Print and shaded views of the part. All mm, measured from the part's lowest x, y and z. Round coordinates to 2 decimals unless told otherwise and drop trailing zeros. Loops run counter-clockwise (first coordinate to the right, second up) from the corner with the lowest first, then second, coordinate; pieces in that order, holes last. Notation, with made-up numbers: (8, -13.75) -> (64, -13.75) arc R25 cw to (64, 6.25) -> close; hole circle Ø2 at (-33, 22). An arc over 180 degrees is marked (long way). Answer as CSV lines item,"result".
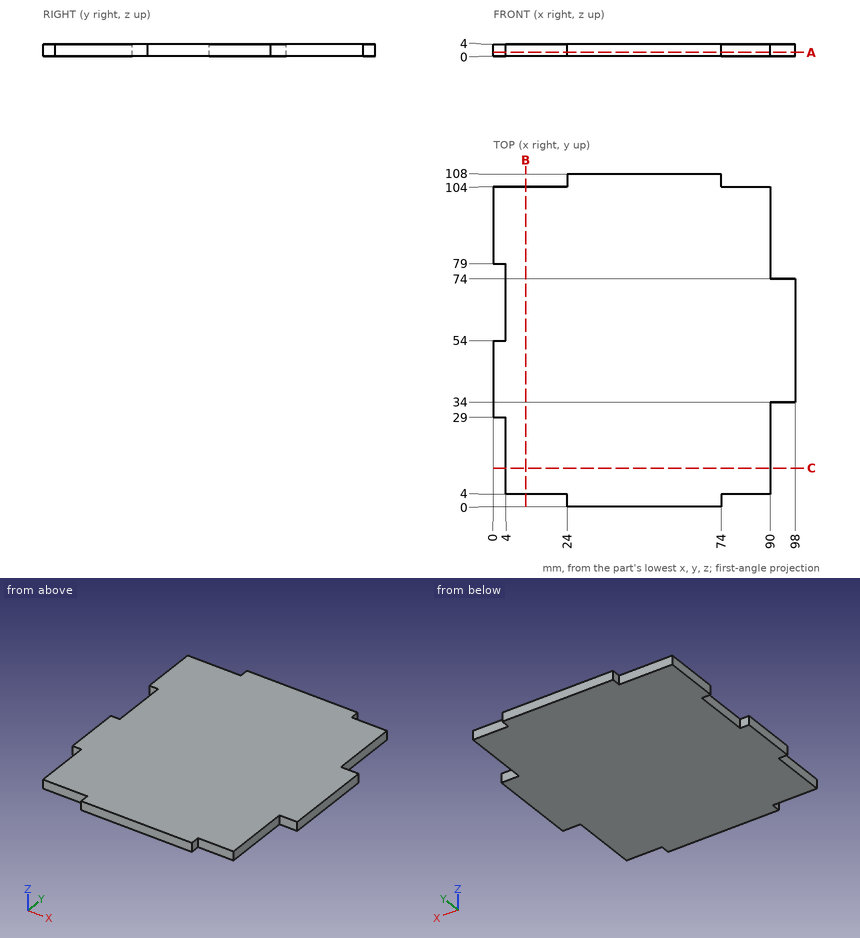
Q1. Slice it at C-C, the plane y = 12.5. Give the cut face in (x, z), and give its area (3 significant figures).
Results:
outline,"(4, 0) -> (90, 0) -> (90, 4) -> (4, 4) -> close"
area,"344 mm2"
Q2. Drop flat-ended pins along their axis: pin 1 Ø10 at (x, y) = (62, 78.5) entering from -Z; pin 2 Ø1.2 at (x, z) = (1, 1.5) entering from -Y; pin 3 Ø1.2 at (y, z) = (2.5, 1.5) entering from -X; pin 4 Ø2 at (x, z) = (78.5, 2) entering from -Y. Give the stop position or say it passes through.
Results:
pin 1,"z = 0"
pin 2,"y = 29"
pin 3,"x = 24"
pin 4,"y = 4"
Q3. Slice it at B-B, the plane x = 10.5. Give the cut face in (y, z), and give its area (3 significant figures).
Results:
outline,"(4, 0) -> (104, 0) -> (104, 4) -> (4, 4) -> close"
area,"400 mm2"
Q4. Slice it at A-A, the plane z = 1.25. Give the cut face in (x, y), and give its area (3 significant figures).
Results:
outline,"(0, 29) -> (4, 29) -> (4, 4) -> (24, 4) -> (24, 0) -> (74, 0) -> (74, 4) -> (90, 4) -> (90, 34) -> (98, 34) -> (98, 74) -> (90, 74) -> (90, 104) -> (74, 104) -> (74, 108) -> (24, 108) -> (24, 104) -> (0, 104) -> (0, 79) -> (4, 79) -> (4, 54) -> (0, 54) -> close"
area,"9,520 mm2"
Q5. Probe L1, parallel to X at y = 22, z = 3.85; L2, parallel to Y at x = 83, z = 3.05; L3, parallel to X at y = 103.5, z = 2.65. List the from-to ranges inside material, lowest first. Write a range as [from, to].
Results:
L1,"[4, 90]"
L2,"[4, 104]"
L3,"[0, 90]"
